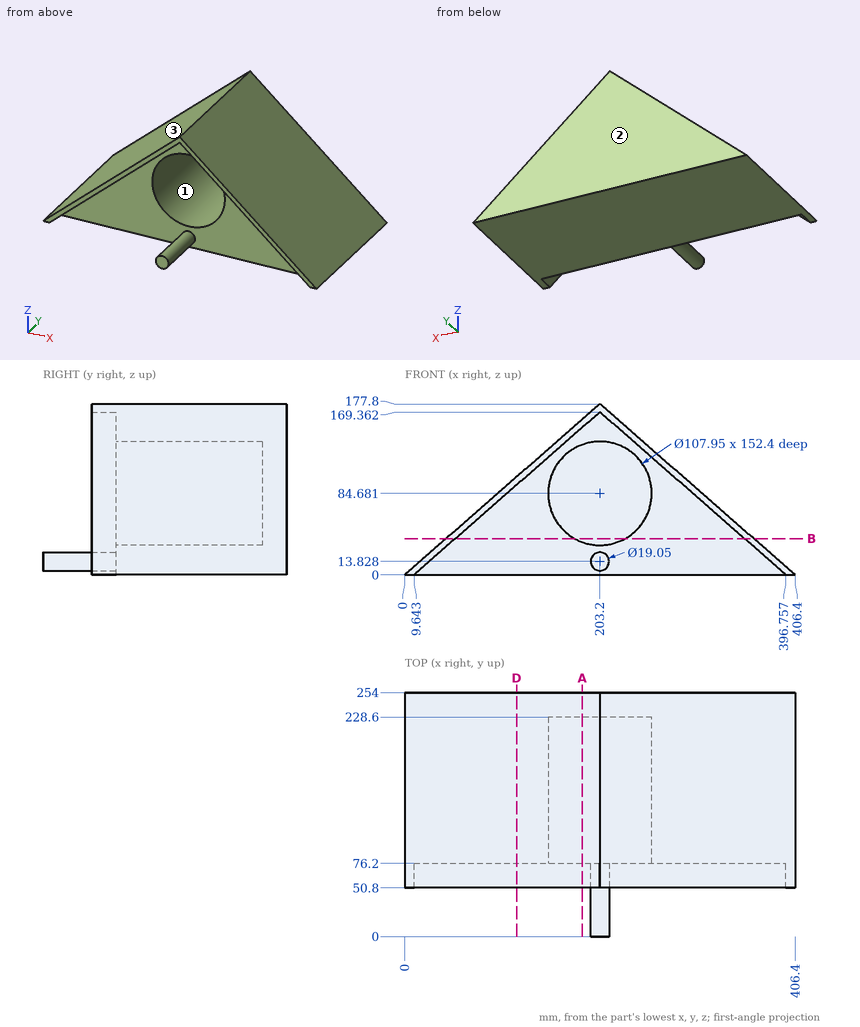
Design review of the part shown in the three views and the two pictorial views. Dimensions are in mm from the part's minimum x, y and z. Coordinates: 2 decimals unless noted, no trailing zeros. Loops run counter-clockwise (first coordinate to the right, second up) from the corner with the lowest first, then second, coordinate; pieces in that order, holes last.
(1) Insertion check: P1, Ø8, axis at y = 130.5, z = 28.5, coming from the +X side; P2, Ø4, axis at x = 194.5, y = 192, coming from the +Z side; P3, Ø1, axis at x = 247.5, y = 221.5, coming from the +Z side (1 decimal). Each pin has a flat end and moves straight along its axis. Give the tip position at first contact, or say it passes through.
Determined:
P1: stops at x = 378.4
P2: stops at z = 171.94
P3: stops at z = 139.5
(2) Consider section D-D, the plane x = 116.5. Give the boundary of the cut face in (y, z).
Determined:
outline: (50.8, 93.5) - (76.2, 93.5) - (76.2, 0) - (254, 0) - (254, 101.94) - (50.8, 101.94) - close
(3) Draft analysis for pull direction X (two halves, no side actions). For the marked faces 1, 2 and 3, state which applies: +X half, -X half, draft (parallel to the pull), parting line (faces both ways), or undercut.
Determined:
face 1: undercut
face 2: draft
face 3: -X half
(4) Consider section B-B, the plane z = 37.5. Give the boundary of the cut face in (x, y) (1 decimal).
Determined:
outline: (42.9, 50.8) - (52.5, 50.8) - (52.5, 76.2) - (177, 76.2) - (177, 228.6) - (229.4, 228.6) - (229.4, 76.2) - (353.9, 76.2) - (353.9, 50.8) - (363.5, 50.8) - (363.5, 254) - (42.9, 254) - close
(5) Wall thickness on L1, parallel to Z at x = 203.2, y = 197.5 (1 decimal); L2, parallel to Y at x = 213, z = 23; L3, parallel to X at y = 228.5, z = 118.5 (1 decimal): over which ranges is each line inside the solid? List them lowest first.
Determined:
L1: z = 0 to 30.7, 138.7 to 177.8
L2: y = 76.2 to 254
L3: x = 135.4 to 161.1, 245.3 to 271
(6) Consider section A-A, the plane x = 185. Give the boundary of the cut face in (y, z) (1 decimal), plus the area to 3 significant figures.
Determined:
outline: (50.8, 153.4) - (76.2, 153.4) - (76.2, 135.5) - (228.6, 135.5) - (228.6, 33.9) - (76.2, 33.9) - (76.2, 0) - (254, 0) - (254, 161.9) - (50.8, 161.9) - close
area: 13,500 mm2
